Geometry: see drawing. Coordinates: mm, zero at the bounding-box minimum. Coordinates: 2 decimals unless noted, no trailing zeros. Order: outer loops, then holes, each group sorted by start corner. A loop starts at its lowest first (then second) coordinate and runs counter-clockwise, first axis right, second up. Notation, with made-up numbers: (-7, 7) -> (16, 7) arc R14 ccw to (16, 30) -> close; hole circle Ø7 at (56, 36). An arc over 180 degrees is marked (long way). Write each question's results on one line, items separated by ' | '.
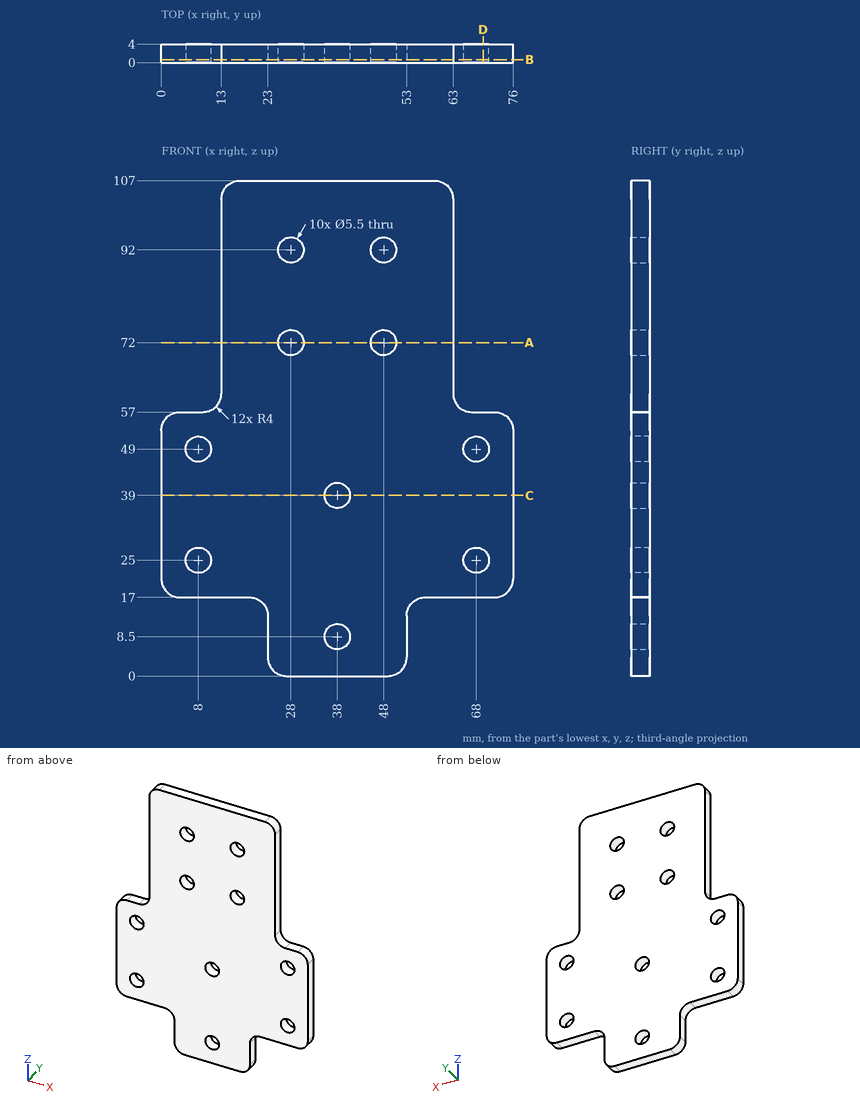
(1) Cut plane C-C, the plane z = 39. Return loops of the section in (x, y), plus the area to 3 significant figures.
Return value:
outline: (0, 0) -> (35.25, 0) -> (35.25, 4) -> (0, 4) -> close; (40.75, 0) -> (76, 0) -> (76, 4) -> (40.75, 4) -> close | area: 282 mm2
(2) Cut plane B-B, the plane y = 0.6. Count the separate pieces of the cut face and the enclosed holes in it, plus the area to 3 significant figures.
Return value:
separate pieces: 1 | enclosed holes: 10 | area: 5,800 mm2
(3) Cut plane D-D, the plane x = 69.5. Return loops of the section in (y, z).
Return value:
outline: (0, 17) -> (4, 17) -> (4, 22.7) -> (0, 22.7) -> close; (0, 27.3) -> (4, 27.3) -> (4, 46.7) -> (0, 46.7) -> close; (0, 51.3) -> (4, 51.3) -> (4, 57) -> (0, 57) -> close
(4) Line query: line 1 along X through (y, z) = (2.75, 92); line 2 along Z through (x, y) = (8, 1.75); line 3 along Z through (x, y) = (38, 2.4). Output: solid intervals per line, ascending. Write a range as from..to.
Return value:
line 1: 13..25.25, 30.75..45.25, 50.75..63 | line 2: 17..22.25, 27.75..46.25, 51.75..57 | line 3: 0..5.75, 11.25..36.25, 41.75..107
(5) Cut plane A-A, the plane z = 72. Return loops of the section in (x, y), plus the area to 3 significant figures.
Return value:
outline: (13, 0) -> (25.25, 0) -> (25.25, 4) -> (13, 4) -> close; (30.75, 0) -> (45.25, 0) -> (45.25, 4) -> (30.75, 4) -> close; (50.75, 0) -> (63, 0) -> (63, 4) -> (50.75, 4) -> close | area: 156 mm2
(6) Pin query (flat end, axial travel): P1, Ø1.2, axis at x = 69, y = 3, coming from the +Z side; P2, Ø9, axis at x = 8, z = 49, coming from the -Y side; P3, Ø5, axis at x = 38, z = 39, coming from the -Y side; P4, Ø1.2, axis at x = 9, y = 2, coming from the -Z side. Return the tip coordinate at first contact, or that it passes through.
Return value:
P1: z = 57 | P2: y = 0 | P3: through | P4: z = 17
